```python
from build123d import *

# Parameters (mm, degrees)
F0_W     = 7.366
F0_H     = 15.24
F1_DEPTH = 6.35


with BuildPart() as f1:
    # F0 (on Top) → F1 (new body)
    with BuildSketch(Plane.XY):
        Polygon((108.494151, 76.2), (-69.305849, 76.2), (-76.671849, 76.2), (-83.021849, 76.2), (-83.021849, -60.96), (-76.671849, -60.96), (-69.305849, -60.96), (108.459485, -60.96), (114.844151, -60.96), (114.844151, -45.72), (108.494151, -45.72), (108.494151, -30.48), (114.844151, -30.48), (114.844151, -15.24), (108.494151, -15.24), (108.494151, 0), (114.844151, 0), (114.844151, 15.24), (108.494151, 15.24), (108.494151, 30.48), (114.844151, 30.48), (114.844151, 45.72), (108.494151, 45.72), (108.494151, 60.96), (114.844151, 60.96), (114.844151, 76.2), align=None)
        with Locations((-72.988849, -38.1)):
            Rectangle(F0_W, F0_H, mode=Mode.SUBTRACT)
        with Locations((-72.988849, -7.62)):
            Rectangle(F0_W, F0_H, mode=Mode.SUBTRACT)
        with Locations((-72.988849, 22.86)):
            Rectangle(F0_W, F0_H, mode=Mode.SUBTRACT)
        with Locations((-72.988849, 53.34)):
            Rectangle(F0_W, F0_H, mode=Mode.SUBTRACT)
    extrude(amount=F1_DEPTH)


solid = f1.part
```
For this review, take the finished solid that the model builds, in its own axes (mm). A direction names the side the tool comes from. Round coordinates to 2 decimals unless told otherwise and drop trailing zeros. Write each loop counter-clockwise with the first axis right and the second up, starting at its lowest first coordinate (ties: lowest second). Pieces come first, ordered by that corner, then holes. Notation, with made-up numbers: (7, 76) - (25, 76) arc R20 ccw to (25, 95) - close; hole circle Ø5 at (29, 60.5). An arc over 180 degrees is marked (long way). Answer as CSV lines item,"result". Start each with the question number.
(1) Add section B-B, the plane z = 2. State how many separate pieces and enclosed holes the cut face has, plus the area to 3 significant figures.
(2) Add section A-A, the plane y = 50.5. State the section outline as (x, z) points.
(3) Mouldability with a two-part tool opening along Y and no side actions: class faces 4 (the flat face through (114.844, 68, 3)), 5 (the flat face through (15, -60.96, 3)), 6 (the flat face through (-73, 15.24, 3)) as +Y half, -Y half, draft (parallel to the pull), parting line (faces both ways), or undercut.
(4) For line 1 (X direction, y = -31, z = 3), list the stretches that pass through material, from the lowest coordinate up.
(5) For pin 1 (1.9 mm diameter, centred on y = -39.5, z = 3, fed in from +X), flat-tipped, find the tip position at first contact; note if it passes through.
(6) Machinability: for faces 1 (the flat face through (-73, 30.48, 3)), 2 (the flat face through (114.844, 38, 3)), 3 (the flat face through (112, 30.48, 3)), which of the approach directions +Z, -Z, +X, -X, +Y, -Y give a long, thin tool a straight path to every point of the face, cutting with its end or side? Answer none if there is none.
From the geometry:
1,separate pieces,"1"
1,enclosed holes,"4"
1,area,"26,300 mm²"
2,outline,"(-83.02, 0) - (-76.67, 0) - (-76.67, 6.35) - (-83.02, 6.35) - close; (-69.31, 0) - (108.49, 0) - (108.49, 6.35) - (-69.31, 6.35) - close"
3,face 4,"draft"
3,face 5,"-Y half"
3,face 6,"undercut"
4,line 1,"x = -83.02 to -76.67, -69.31 to 108.49"
5,pin 1,"stops at x = 108.49"
6,face 1,"+Z, -Z"
6,face 2,"+Z, -Z, +X, +Y, -Y"
6,face 3,"+Z, -Z, +X"
